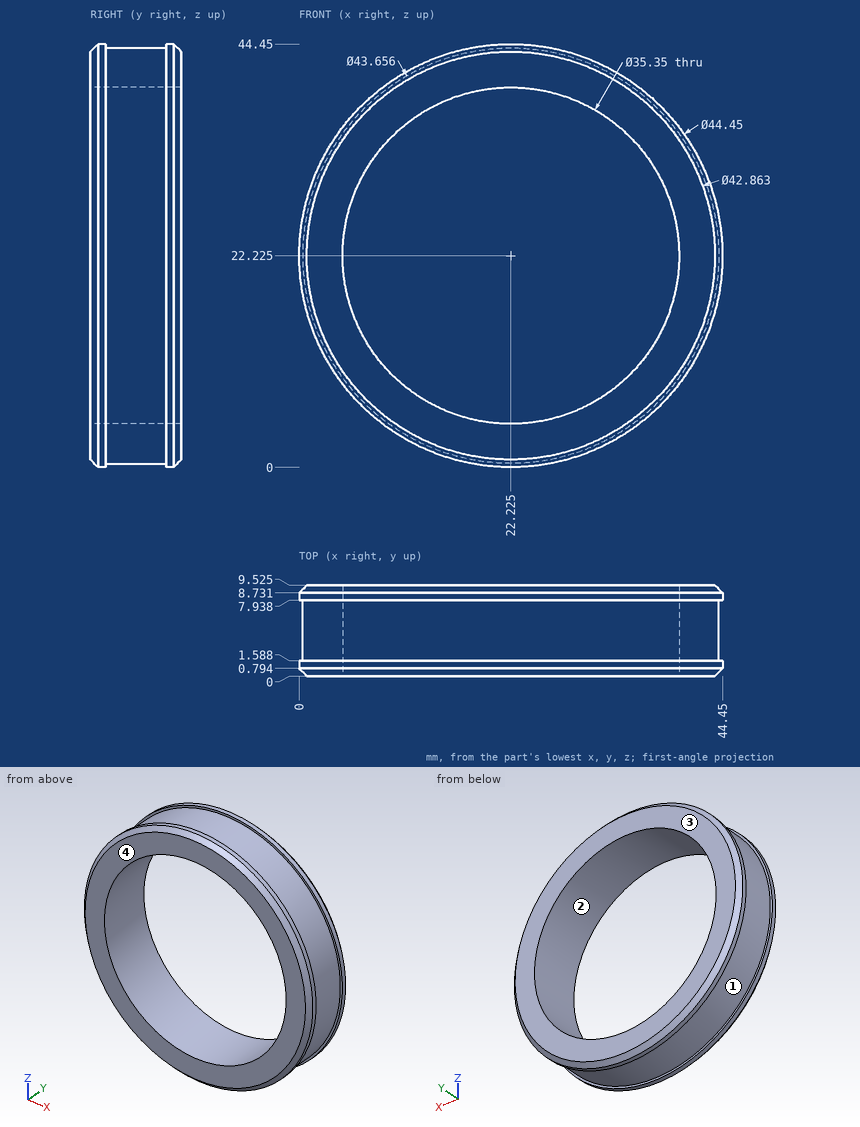
Geometry check sheet. Reference: drawing and pictorial views, mm from the part's lowest x, y, z. Coordinates: 2 decimals unless noted, no trailing zeros. Write item = value, one per line.
Q1. Mould release check, pull along Y, two halves, no side actions. Record for the marked faces 1, 2, 3 and 4: released by +Y, released by -Y, zero draft, split by the parting line, or undercut.
Answer:
face_1 = undercut
face_2 = zero draft
face_3 = released by +Y
face_4 = released by -Y
Q2. Material ranges on L1, parallel to Z at x = 18, y = 8.75 (1 decimal); L2, parallel to X at y = 2.25, z = 31; L3, parallel to X at y = 2.5, z = 19, recorded low to high. Write a range as from..to.
Answer:
L1 = 0.4..5.1, 39.4..44
L2 = 2.24..6.88, 37.57..42.21
L3 = 0.64..4.85, 39.6..43.81
Q3. Go/stop test with flat-tipped pins: pin 1 Ø1 at (y, z) = (5, 30.5) entering from +X; pin 2 Ø2 at (x, y) = (9, 3) entering from -Z; pin 3 Ø1.5 at (y, z) = (5, 33.5) entering from +X. Record where each tip stops, or that it passes through.
Answer:
pin_1 = 42.62
pin_2 = 4.14
pin_3 = 41.35
